The drawing under review shows one solid part. Ordinate dimensions are in mm from its lowest x, y, z. Round coordinates to 2 decimals unless told otherwise and drop trailing zeros. Order: outer loops, then holes, each group sorted by start corner. A loop starts at its lowest first (then second) coordinate and runs counter-clockwise, first axis right, second up. Notation, with made-up numbers: (89, 18) - (123, 18) arc R29 cw to (123, 50) - close; hole circle Ø4 at (71, 88). An arc over 180 degrees is marked (long way). Answer as a JSON object with one key per item and string values. Group by question number.
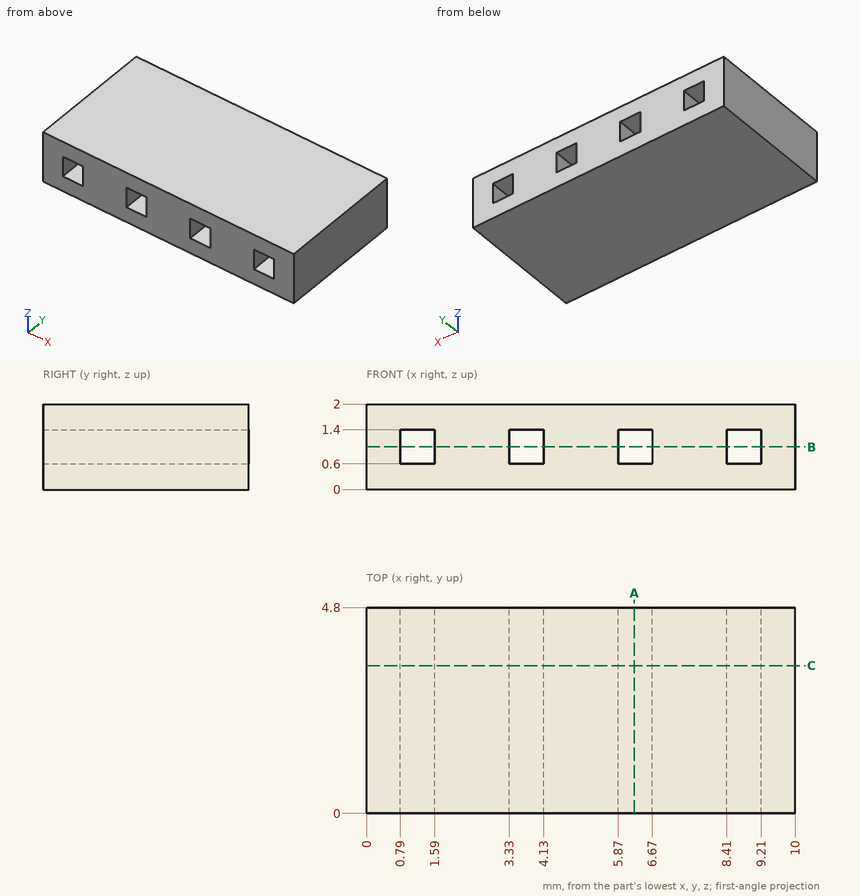
1. Take a section at B-B, the plane z = 1. Give the boundary of the cut face in (x, y).
2. Take a section at C-C, the plane y = 3.45. Give the boundary of the cut face in (x, z), then the cut area to 3 significant figures.
3. Take a section at A-A, the plane x = 6.25. Give the boundary of the cut face in (y, z).
4. To check wall thickness, follow line 1 (X direction, y = 0.5, z = 0.85); line 2 (Z direction, x = 9, y = 3.75). State the ranges of each line that lie inside material, in increasing order. Write a range as from..to.
Response values:
{
 "1": {"outline": "(0, 0) - (0.79, 0) - (0.79, 4.8) - (0, 4.8) - close; (1.59, 0) - (3.33, 0) - (3.33, 4.8) - (1.59, 4.8) - close; (4.13, 0) - (5.87, 0) - (5.87, 4.8) - (4.13, 4.8) - close; (6.67, 0) - (8.41, 0) - (8.41, 4.8) - (6.67, 4.8) - close; (9.21, 0) - (10, 0) - (10, 4.8) - (9.21, 4.8) - close"},
 "2": {"outline": "(0, 0) - (10, 0) - (10, 2) - (0, 2) - close; hole (0.79, 0.6) - (1.59, 0.6) - (1.59, 1.4) - (0.79, 1.4) - close; hole (3.33, 0.6) - (4.13, 0.6) - (4.13, 1.4) - (3.33, 1.4) - close; hole (5.87, 0.6) - (6.67, 0.6) - (6.67, 1.4) - (5.87, 1.4) - close; hole (8.41, 0.6) - (9.21, 0.6) - (9.21, 1.4) - (8.41, 1.4) - close", "area": "17.4 mm2"},
 "3": {"outline": "(0, 0) - (4.8, 0) - (4.8, 0.6) - (0, 0.6) - close; (0, 1.4) - (4.8, 1.4) - (4.8, 2) - (0, 2) - close"},
 "4": {"line 1": "0..0.79, 1.59..3.33, 4.13..5.87, 6.67..8.41, 9.21..10", "line 2": "0..0.6, 1.4..2"}
}
